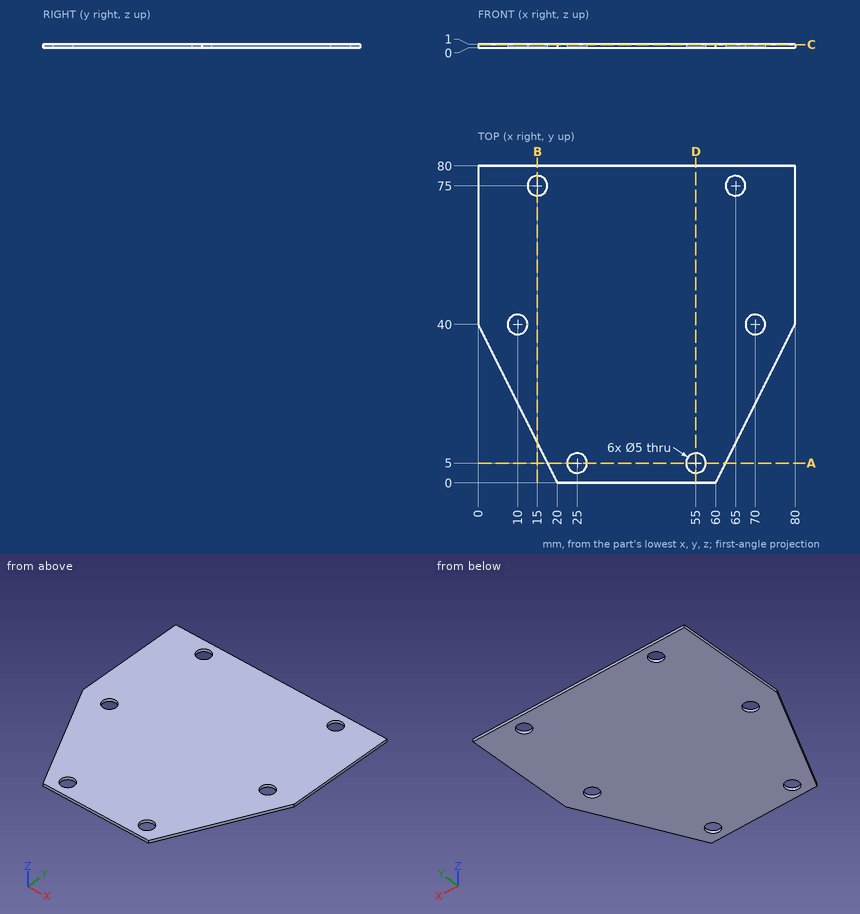
Part print with two shaded views. Sizes in mm from the minimum x, y, z corner. Round coordinates to 2 decimals unless told otherwise and drop trailing zeros. Order: outer loops, then holes, each group sorted by start corner. A loop starts at its lowest first (then second) coordinate and runs counter-clockwise, first axis right, second up. Notation, with made-up numbers: M 81,59 L 126,59 A15 ccw 126,82 Z; hole C 28.25,-8 d7. An arc over 180 degrees is marked long. Use CSV: the item, a comma, the result in double quotes. Start each with the question number.
(1) Flat gauge pin, fed straight in: P1, Ø3, axis at x = 70, y = 40, coming from the -Z side. Where does the tip first touch, or does it go through?
(2) Cut at B-B on x = 15. List the corners of the cut face in (y, z).
(3) Cut at D-D on x = 55. List the corners of the cut face in (y, z).
(4) Cut at C-C on z = 0.85. List the corners of the cut face in (x, y).
(5) Cut at A-A on y = 5. List the corners of the cut face in (x, z).
(6) Drill centre lines: probe 1 along Y at (x, z) = (10, 0.7); probe 2 along Y at (x, z) = (55, 0.8); probe 3 along X at (y, z) = (9, 0.65). Where is each one in solid material? Low to high.
Findings:
1,P1,"passes through"
2,outline,"M 10,0 L 72.5,0 L 72.5,1 L 10,1 Z; M 77.5,0 L 80,0 L 80,1 L 77.5,1 Z"
3,outline,"M 0,0 L 2.5,0 L 2.5,1 L 0,1 Z; M 7.5,0 L 80,0 L 80,1 L 7.5,1 Z"
4,outline,"M 0,40 L 20,0 L 60,0 L 80,40 L 80,80 L 0,80 Z; hole C 10,40 d5; hole C 15,75 d5; hole C 25,5 d5; hole C 55,5 d5; hole C 65,75 d5; hole C 70,40 d5"
5,outline,"M 17.5,0 L 22.5,0 L 22.5,1 L 17.5,1 Z; M 27.5,0 L 52.5,0 L 52.5,1 L 27.5,1 Z; M 57.5,0 L 62.5,0 L 62.5,1 L 57.5,1 Z"
6,probe 1,"y = 20 to 37.5, 42.5 to 80"
6,probe 2,"y = 0 to 2.5, 7.5 to 80"
6,probe 3,"x = 15.5 to 64.5"
